Answer from the drawing. Dimensions are ordinates in mm from the lowest x, y and z of the part. A direction names the side the tool comes from. Give positions to 0.01 mm unless a question says otherwise; leave off trailing zeros. Loops run counter-clockwise (first coordinate to the right, second up) from the corner with the lowest first, then second, coordinate; pieces in that order, holes last.
Item 1: Consider line 1 along Y through (x, z) = (27, 3); line 2 along Y through (x, z) = (28, 5.45); line 3 along X through (y, z) = (8.5, 4.55). Determine where each line is inside the solid, lowest interval first.
Item 2: Section B-B, the plane z = 3 is taken. Give the vertices of the cut face in (x, y), and give its area (3 significant figures).
Item 3: Section A-A, the plane x = 6 is taken. Give the vertices of the cut face in (y, z).
Item 4: Each of these flat-tipped pins is pushed along its axis until it touches: pin 1 Ø3 at (x, z) = (15.5, 2.5) entering from -Y; pin 2 Ø3 at (x, z) = (17.5, 2) entering from +Y. Where does it stop, or does it pass through?
Item 5: Section D-D, the plane x = 25.5 is taken. Give the vertices of the cut face in (y, z).
Item 6: Section C-C, the plane y = 6 is taken. Give the vertices of the cut face in (x, z), and give its area (3 significant figures).
Item 7: The mould has two halves that part along X. Classify the marked faces 4, 5 and 6: pulls with the +X half, pulls with the -X half, needs draft (parallel to the pull), parting line crosses it, or undercut.
Item 8: A tool of negligible diameter and unlimited length cuts with its end or side. For the marked faces 1, 2 and 3, from which of +Z, -Z, +X, -X, +Y, -Y can it reach the whole face along a straight path? Write none if from no direction.
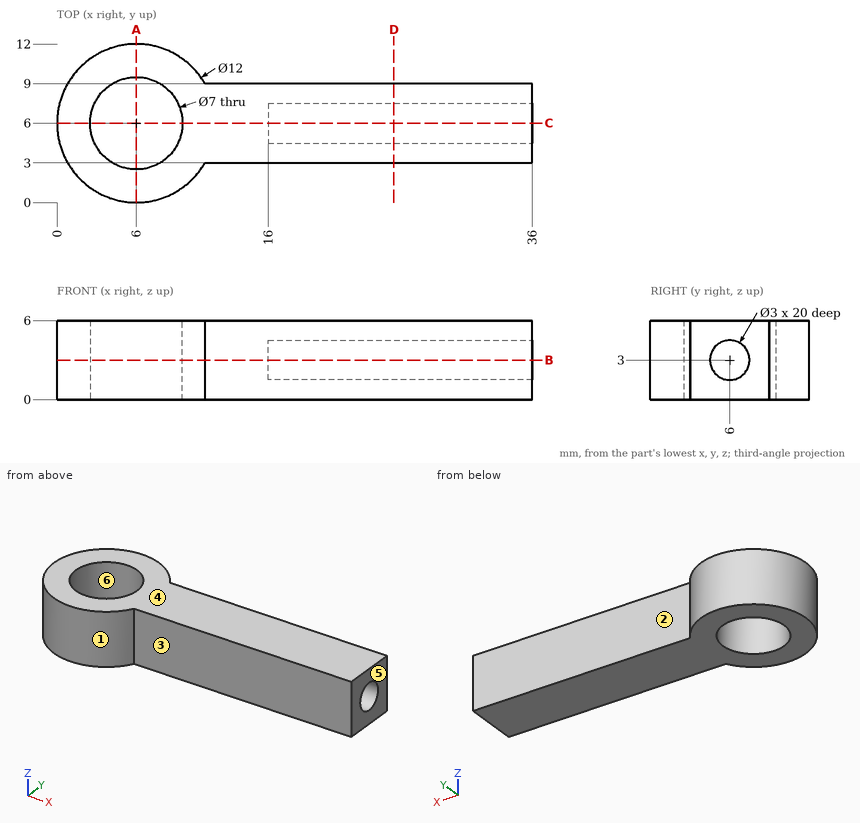
Worked answers:
1. line 1: y = 3 to 4.5, 7.5 to 9
1. line 2: y = 3 to 9
1. line 3: x = 0.55 to 3.55, 8.45 to 36
2. outline: (11.2, 3) - (36, 3) - (36, 4.5) - (16, 4.5) - (16, 7.5) - (36, 7.5) - (36, 9) - (11.2, 9) arc R6 ccw (long way) to start; hole circle Ø7 at (6, 6)
2. area: 160 mm2
3. outline: (0, 0) - (2.5, 0) - (2.5, 6) - (0, 6) - close; (9.5, 0) - (12, 0) - (12, 6) - (9.5, 6) - close
4. pin 1: stops at y = 3
4. pin 2: stops at y = 9
5. outline: (3, 0) - (9, 0) - (9, 6) - (3, 6) - close; hole circle Ø3 at (6, 3)
6. outline: (0, 0) - (2.5, 0) - (2.5, 6) - (0, 6) - close; (9.5, 0) - (36, 0) - (36, 1.5) - (16, 1.5) - (16, 4.5) - (36, 4.5) - (36, 6) - (9.5, 6) - close
6. area: 114 mm2
7. face 4: needs draft
7. face 5: pulls with the +X half
7. face 6: undercut
8. face 1: +Z, -Z
8. face 2: +Z, -Z, +X, +Y
8. face 3: +Z, -Z, +X, -Y
